from build123d import *

# Parameters (mm, degrees)
SKETCH1_R           = 77.4600051
BOSS_EXTRUDE1_DEPTH = 3.175
SKETCH20_R          = 22.86
SKETCH20_R_2        = 2.0193
CUT_EXTRUDE10_DEPTH = 250.596695835
CUT_EXTRUDE11_DEPTH = 3.175
SKETCH22_R          = 2.0193
CUT_EXTRUDE12_DEPTH = 250.596695835
CUT_EXTRUDE13_DEPTH = 250.596695835


with BuildPart() as part:
    # Sketch1 → Boss-Extrude1 (new body)
    with BuildSketch(Plane(origin=(0, 0, 0), x_dir=(1, 0, 0), z_dir=(0, 1, 0))):
        with Locations(Location((0, 0, 0), (0, 0, 270))):
            Circle(SKETCH1_R)
    extrude(amount=BOSS_EXTRUDE1_DEPTH)

    # Sketch20 → Cut-Extrude10 (cut, through all)
    with BuildSketch(Plane(origin=(-73.768816189, 3.175, -121.080352405), x_dir=(1, 0, 0), z_dir=(0, 1, 0))):
        with Locations(Location((73.768816189, -121.080352405, 0), (0, 0, 270))):
            Circle(SKETCH20_R)
        with Locations(Location((73.768816189, -88.060352405, 0), (0, 0, 270))):
            Circle(SKETCH20_R_2)
        with Locations(Location((106.788816189, -121.080352405, 0), (0, 0, 270))):
            Circle(SKETCH20_R_2)
        with Locations(Location((73.768816189, -154.100352405, 0), (0, 0, 270))):
            Circle(SKETCH20_R_2)
        with Locations(Location((40.748816189, -121.080352405, 0), (0, 0, 270))):
            Circle(SKETCH20_R_2)
    extrude(amount=-CUT_EXTRUDE10_DEPTH, mode=Mode.SUBTRACT)

    # Sketch21 → Cut-Extrude11 (cut)
    with BuildSketch(Plane(origin=(-73.768816189, 3.175, -121.080352405), x_dir=(1, 0, 0), z_dir=(0, 1, 0))):
        with BuildLine():
            Line((41.420818538, -92.324457203), (32.440562417, -83.344201082))
            ThreePointArc((32.440562417, -83.344201082), (32.440562417, -79.752098633), (36.032664865, -79.752098633))
            Line((36.032664865, -79.752098633), (45.012920986, -88.732354754))
            ThreePointArc((45.012920986, -88.732354754), (45.012920986, -92.324457203), (41.420818538, -92.324457203))
        make_face()
    extrude(amount=-CUT_EXTRUDE11_DEPTH, mode=Mode.SUBTRACT)

    # Sketch22 → Cut-Extrude12 (cut, through all)
    with BuildSketch(Plane(origin=(-73.768816189, 3.175, -121.080352405), x_dir=(1, 0, 0), z_dir=(0, 1, 0))):
        with Locations(Location((48.605023435, -95.916559651, 0), (0, 0, 270))):
            Circle(SKETCH22_R)
    extrude(amount=-CUT_EXTRUDE12_DEPTH, mode=Mode.SUBTRACT)

    # Sketch23 → Cut-Extrude13 (cut, through all)
    with BuildSketch(Plane(origin=(-73.768816189, 3.175, -121.080352405), x_dir=(1, 0, 0), z_dir=(0, 1, 0))):
        with BuildLine():
            ThreePointArc((34.405967979, -136.122213123), (36.00963526, -139.786919397), (37.953573181, -143.283049568))
            ThreePointArc((37.953573181, -143.283049568), (46.974494303, -145.399596657), (49.091041391, -136.378675534))
            ThreePointArc((49.091041391, -136.378675534), (47.751609959, -133.969737166), (46.646635186, -131.444644817))
            ThreePointArc((46.646635186, -131.444644817), (38.18751743, -127.663095366), (34.405967979, -136.122213123))
        make_face()
    extrude(amount=-CUT_EXTRUDE13_DEPTH, mode=Mode.SUBTRACT)


solid = part.part
Verification items for the finished model (mm, model axes). A direction names the side the tool comes from. Coordinates: 2 decimals unless noted, no trailing zeros. Loops run counter-clockwise (first coordinate to the right, second up) from the corner with the lowest first, then second, coordinate; pieces in that order, holes last. Notation, with made-up numbers: (-17, 72.5) -> (27, 72.5) arc R23 cw to (27, 85.5) -> close; hole circle Ø9 at (67, 26.5). An arc over 180 degrees is marked (long way). Write each question's results on one line, items separated by ' | '.
Item 1: Gauge pin test, flat ends, axial feed: pin 1 (1 mm diameter, centred on x = 34, y = 0.5, fed in from -Z); pin 2 (4.5 mm diameter, centred on x = 0, z = 33.02, fed in from +Y) (3 decimals); pin 3 (1 mm diameter, centred on x = 29, y = 1, fed in from +Z); pin 4 (3 mm diameter, centred on x = 33.02, z = 0, fed in from +Y). Record the tip position at first contact, or that the pin passes through.
Found:
pin 1: stops at z = -69.84 | pin 2: stops at y = 3.175 | pin 3: stops at z = 72.03 | pin 4: passes through
Item 2: Section check D-D, the plane z = 33.02. Enter the section's corners in (x, y) (3 decimals), plus the area to 3 significant figures.
Found:
outline: (-70.069, 0) -> (-2.019, 0) -> (-2.019, 3.175) -> (-70.069, 3.175) -> close; (2.019, 0) -> (70.069, 0) -> (70.069, 3.175) -> (2.019, 3.175) -> close | area: 432 mm2
Item 3: Section check A-A, the plane z = 0. Enter the section's corners in (x, y) (3 decimals).
Found:
outline: (-77.46, 0) -> (-35.039, 0) -> (-35.039, 3.175) -> (-77.46, 3.175) -> close; (-31.001, 0) -> (-22.86, 0) -> (-22.86, 3.175) -> (-31.001, 3.175) -> close; (22.86, 0) -> (31.001, 0) -> (31.001, 3.175) -> (22.86, 3.175) -> close; (35.039, 0) -> (77.46, 0) -> (77.46, 3.175) -> (35.039, 3.175) -> close
Item 4: Mould release check, pull along Z, two halves, no side actions. Record for faces 1 (the face through (18, 0, 16)), 2 (the face through (22.665, 1.61, -2.976)), 3 (the face through (23.27, 1.57, 73.88)): +Z half, -Z half, draft (parallel to the pull), parting line (faces both ways), or undercut.
Found:
face 1: draft | face 2: undercut | face 3: parting line
Item 5: Section check B-B, the plane x = 0. Enter the section's corners in (y, z) (3 decimals), plus the area to 3 significant figures.
Found:
outline: (0, -77.46) -> (3.175, -77.46) -> (3.175, -35.039) -> (0, -35.039) -> close; (0, -31.001) -> (3.175, -31.001) -> (3.175, -22.86) -> (0, -22.86) -> close; (0, 22.86) -> (3.175, 22.86) -> (3.175, 31.001) -> (0, 31.001) -> close; (0, 35.039) -> (3.175, 35.039) -> (3.175, 77.46) -> (0, 77.46) -> close | area: 321 mm2
Item 6: Tool access check on faces 4 (the face through (18, 3.175, 16)), 5 (the face through (-33.31, 1.61, -36.9)). Record the directions out of +Z, -Z, +X, -X, +Y, -Y that give a thin tool (end or side, any length) a straight path to the whole face; none if there is none.
Found:
face 4: +Z, -Z, +X, -X, +Y | face 5: +Y, -Y
Item 7: Material ranges on L1, parallel to X at y = 2.5, z = 0; L2, parallel to Z at x = -36, y = 1.5; L3, parallel to X at y = 2.5, z = 18.5, recorded low to high.
Found:
L1: x = -77.46 to -35.04, -31 to -22.86, 22.86 to 31, 35.04 to 77.46 | L2: z = -68.59 to -39.59, -32.41 to 6.76, 21.9 to 68.59 | L3: x = -75.22 to -37.86, -23.7 to -13.43, 13.43 to 75.22
Item 8: Section check C-C, the plane y = 1.3. Count the separate pieces of the cut face and the enclosed holes in it, plus the area to 3 significant figures.
Found:
separate pieces: 1 | enclosed holes: 8 | area: 16,800 mm2
